from build123d import *

# Parameters (mm, degrees)
BOSS_EXTRU_1_DEPTH      = 4.35
ENL_V_MAT_EXTRU_1_DEPTH = 38.269393438
CONG_3_R                = 5
ESQUISSE3_R             = 1.5
ENL_V_MAT_EXTRU_2_DEPTH = 38.269393579
BOSS_EXTRU_2_DEPTH      = 4.35


with BuildPart() as part:
    # Esquisse1 → Boss.-Extru.1 (new body)
    with BuildSketch(Plane.XY):
        with BuildLine():
            Line((-13.183298291, -31.679408844), (-0.713739606, -32.039150948))
            ThreePointArc((-0.713739606, -32.039150948), (13.826896651, 2.211449904), (-6.128687986, 33.616997237))
            ThreePointArc((-6.128687986, 33.616997237), (-12.95399094, 31.768960554), (-11.105954257, 24.9436576))
            ThreePointArc((-11.105954257, 24.9436576), (3.84132079, 1.61453914), (-6.69721834, -24.00982412))
            ThreePointArc((-6.69721834, -24.00982412), (-10.263527106, -27.571231769), (-13.183298291, -31.679408844))
        make_face()
    extrude(amount=BOSS_EXTRU_1_DEPTH)

    # Esquisse2 → Enlèv. mat.-Extru.1 (cut, through all)
    with BuildSketch(Plane(origin=(0, 0, 0), x_dir=(-1, 0, 0), z_dir=(0, 0, -1))):
        with BuildLine():
            Line((13.183298291, -31.679408844), (0.713739606, -32.039150948))
            ThreePointArc((0.713739606, -32.039150948), (5.648573529, -29.472487497), (6.69721834, -24.00982412))
            ThreePointArc((6.69721834, -24.00982412), (10.263527106, -27.571231769), (13.183298291, -31.679408844))
        make_face()
    extrude(amount=-ENL_V_MAT_EXTRU_1_DEPTH, mode=Mode.SUBTRACT)

    # Congé3
    cong_3_edges = [part.edges().sort_by_distance(p)[0] for p in [
        (-0.713739606, -32.039150948, 2.175),
        (-6.69721834, -24.00982412, 2.175),
    ]]
    fillet(cong_3_edges, radius=CONG_3_R - 0.0001)  # a hair under: the kernel refuses the full size

    # Esquisse3 → Enlèv. mat.-Extru.2 (cut, through all)
    with BuildSketch(Plane.XY.offset(4.35)):
        with Locations((-8.617321121, 29.280327419)):
            Circle(ESQUISSE3_R)
        with Locations((8.901780596, 0.257662949)):
            Circle(ESQUISSE3_R)
        with Locations((-2.180082362, -26.639815256)):
            Circle(ESQUISSE3_R)
    extrude(amount=-ENL_V_MAT_EXTRU_2_DEPTH, mode=Mode.SUBTRACT)

    # Esquisse4 → Boss.-Extru.2 (add, through all)
    with BuildSketch(Plane.XY.offset(4.35)):
        with BuildLine():
            Line((-9.822535933, 22.144666991), (-8.891427789, 23.540777623))
            ThreePointArc((-8.891427789, 23.540777623), (-9.983360232, 24.266418144), (-11.105954257, 24.9436576))
            ThreePointArc((-11.105954257, 24.9436576), (-11.749605725, 25.383047193), (-12.317161418, 25.917117378))
            Line((-12.317161418, 25.917117378), (-12.247003841, 25.565996611))
            Line((-12.247003841, 25.565996611), (-11.635101494, 22.503581534))
            ThreePointArc((-11.635101494, 22.503581534), (-10.848728229, 21.718565469), (-9.822535933, 22.144666991))
        make_face()
        with BuildLine():
            Line((-6.720773728, 19.63604394), (-5.602744878, 20.887482618))
            ThreePointArc((-5.602744878, 20.887482618), (-7.081127932, 22.175442131), (-8.640486445, 23.364078822))
            Line((-8.640486445, 23.364078822), (-8.464930853, 20.246068108))
            ThreePointArc((-8.464930853, 20.246068108), (-7.796654849, 19.358351758), (-6.720773728, 19.63604394))
        make_face()
        with BuildLine():
            Line((-4.002247722, 16.716500355), (-2.719479126, 17.798439356))
            ThreePointArc((-2.719479126, 17.798439356), (-4.002235611, 19.281339204), (-5.379119408, 20.677278733))
            Line((-5.379119408, 20.677278733), (-5.643393478, 17.565531668))
            ThreePointArc((-5.643393478, 17.565531668), (-5.106472893, 16.592726743), (-4.002247722, 16.716500355))
        make_face()
        with BuildLine():
            Line((-1.720891689, 13.443958065), (-0.298832635, 14.33493243))
            ThreePointArc((-0.298832635, 14.33493243), (-1.360513504, 15.983352852), (-2.527606113, 17.558900694))
            Line((-2.527606113, 17.558900694), (-3.22646682, 14.515152299))
            ThreePointArc((-3.22646682, 14.515152299), (-2.831553807, 13.476558611), (-1.720891689, 13.443958065))
        make_face()
        with BuildLine():
            Line((0.078033764, 9.883342162), (1.611170559, 10.565675544))
            ThreePointArc((1.611170559, 10.565675544), (0.791628357, 12.346912961), (-0.142518712, 14.07081128))
            Line((-0.142518712, 14.07081128), (-1.262101119, 11.155447526))
            ThreePointArc((-1.262101119, 11.155447526), (-1.017030492, 10.071670094), (0.078033764, 9.883342162))
        make_face()
        with BuildLine():
            Line((1.358839136, 6.105292932), (2.972637242, 6.565448283))
            ThreePointArc((2.972637242, 6.565448283), (2.411492888, 8.444164113), (1.728824224, 10.282211897))
            Line((1.728824224, 10.282211897), (0.210731898, 7.553071689))
            ThreePointArc((0.210731898, 7.553071689), (0.301098098, 6.445611945), (1.358839136, 6.105292932))
        make_face()
        with BuildLine():
            Line((2.096114089, 2.184764392), (3.758556811, 2.413612532))
            ThreePointArc((3.758556811, 2.413612532), (3.46694304, 4.352534286), (3.04929648, 6.268265872))
            Line((3.04929648, 6.268265872), (1.16281219, 3.779493562))
            ThreePointArc((1.16281219, 3.779493562), (1.096681157, 2.670322781), (2.096114089, 2.184764392))
        make_face()
        with BuildLine():
            Line((2.275231572, -1.800462743), (3.953337136, -1.807462011))
            ThreePointArc((3.953337136, -1.807462011), (3.937039374, 0.15319873), (3.792700751, 2.108607261))
            Line((3.792700751, 2.108607261), (1.575251109, -0.090421541))
            ThreePointArc((1.575251109, -0.090421541), (1.35393484, -1.179298138), (2.275231572, -1.800462743))
        make_face()
        with BuildLine():
            Line((0.955923809, -9.649040634), (2.565827278, -10.122641832))
            ThreePointArc((2.565827278, -10.122641832), (3.095663042, -8.234857357), (3.501051982, -6.316494523))
            Line((3.501051982, -6.316494523), (0.759343223, -7.811768298))
            ThreePointArc((0.759343223, -7.811768298), (0.243820453, -8.79607994), (0.955923809, -9.649040634))
        make_face()
        with BuildLine():
            Line((1.89263801, -5.771324181), (3.553113903, -6.014031995))
            ThreePointArc((3.553113903, -6.014031995), (3.812455487, -4.07053049), (3.944288385, -2.114239038))
            Line((3.944288385, -2.114239038), (1.439866137, -3.979897042))
            ThreePointArc((1.439866137, -3.979897042), (1.067755401, -5.026876858), (1.89263801, -5.771324181))
        make_face()
        with BuildLine():
            Line((-0.516327235, -13.356680753), (1.011064381, -14.051779397))
            ThreePointArc((1.011064381, -14.051779397), (1.80088273, -12.257164359), (2.471785062, -10.414789202))
            Line((2.471785062, -10.414789202), (-0.452816504, -11.510013499))
            ThreePointArc((-0.452816504, -11.510013499), (-1.101523675, -12.412128869), (-0.516327235, -13.356680753))
        make_face()
        with BuildLine():
            Line((-2.494906628, -16.820687389), (-1.080329313, -17.723493178))
            ThreePointArc((-1.080329313, -17.723493178), (-0.046197856, -16.057651562), (0.876907606, -14.327815597))
            Line((0.876907606, -14.327815597), (-2.172564591, -15.001261883))
            ThreePointArc((-2.172564591, -15.001261883), (-2.941586238, -15.803283605), (-2.494906628, -16.820687389))
        make_face()
        with BuildLine():
            Line((-4.940560652, -19.972336923), (-3.666861923, -21.064938782))
            ThreePointArc((-3.666861923, -21.064938782), (-2.40893385, -19.560919792), (-1.251939064, -17.977941831))
            Line((-1.251939064, -17.977941831), (-4.365782364, -18.216249374))
            ThreePointArc((-4.365782364, -18.216249374), (-5.239861602, -18.902265862), (-4.940560652, -19.972336923))
        make_face()
        with BuildLine():
            ThreePointArc((-5.229503112, -22.686931264), (-4.539706777, -22.000844712), (-3.872520027, -21.292751794))
            Line((-3.872520027, -21.292751794), (-6.988957821, -21.091192728))
            ThreePointArc((-6.988957821, -21.091192728), (-7.95075349, -21.647593865), (-7.804769136, -22.749102695))
            Line((-7.804769136, -22.749102695), (-6.69721834, -24.00982412))
            ThreePointArc((-6.69721834, -24.00982412), (-5.952466431, -23.360464628), (-5.229503112, -22.686931264))
        make_face()
    extrude(amount=-BOSS_EXTRU_2_DEPTH)


solid = part.part
Model file for the job. Use its own axes, mm. A direction names the side the tool comes from. Give positions to 0.01 mm unless a question says otherwise; leave off trailing zeros. Order: outer loops, then holes, each group sorted by start corner. A loop starts at its lowest first (then second) coordinate and runs counter-clockwise, first axis right, second up. Notation, with made-up numbers: (16.25, 56.5) - (44.25, 56.5) arc R20 ccw to (44.25, 88.5) - close; hole circle Ø2 at (77.25, 43.25). An arc over 180 degrees is marked (long way). Write item = value, one per line. Start each with the question number.
1. Which spindle directions (+Z, -Z, +X, -X, +Y, -Y) get a long thin tool onto all of the face, cutting with end or side? Do faces 4 (the flat face through (0.98, 8.94, 2.21)), 5 (the flat face through (1.75, -9.883, 2.205)). Say none if no direction does.
2. Drop flat-ended pins along their axis: P1, Ø1.5, axis at x = 0, z = 2, coming from the +Y side; P2, Ø6, axis at x = 9.5, y = 21.5, coming from the +Z side; P3, Ø2, axis at x = -10, z = 1.5, coming from the +Y side; P4, Ø2.5, axis at x = 8.9, y = 0.26, coming from the +Z side. Give the stop position or say it passes through.
3. Two-plate mould, pull along Y, no slides. Class faces 1 (the flat face through (6, 2, 4.35)), 2 (the cylindrical face through (-1.029, 10.083, 2.205)), 3 (the cylindrical face through (13.72, 3.31, 2.14)): pulls with the +Y half, pulls with the -Y half, needs draft (parallel to the pull), parting line crosses it, or undercut.
4. Cut at A-A, the plane x = 9. List the corners of the cut face in (y, z), and give its area (3 significant figures).
5. Cut at D-D, the plane y = -7. List the corners of the cut face in (x, z), and give its area (3 significant figures).
6. Cut at B-B, the plane y = 30. List the corners of the cut face in (x, z), and give its area (3 significant figures).
7. Cut at C-C, the plane z = 2.5. State how many separate pieces and enclosed holes the cut face has, and give its area (3 significant figures).
8. Probe line 1 along Y through (x, z) = (-5, 1.85); line 2 along Y through (x, z) = (0.5, 0.8); line 3 along X through (y, z) = (10.5, 1.15). List the from-to ranges inside material, lowest first.
Taken from the geometry:
q1.face_4 = +Z, -Z
q1.face_5 = +Z, -Z, -X
q2.P1 = 29.92
q2.P2 = 4.35
q2.P3 = 34.27
q2.P4 = through
q3.face_1 = needs draft
q3.face_2 = undercut
q3.face_3 = parting line crosses it
q4.outline = (-20.37, 0) - (-1.24, 0) - (-1.24, 4.35) - (-20.37, 4.35) - close; (1.75, 0) - (18.22, 0) - (18.22, 4.35) - (1.75, 4.35) - close
q4.area = 155 mm²
q5.outline = (2.25, 0) - (13.52, 0) - (13.52, 4.35) - (2.25, 4.35) - close
q5.area = 49.0 mm²
q6.outline = (-13.57, 0) - (-9.93, 0) - (-9.93, 4.35) - (-13.57, 4.35) - close; (-7.3, 0) - (-0.85, 0) - (-0.85, 4.35) - (-7.3, 4.35) - close
q6.area = 43.8 mm²
q7.separate_pieces = 1
q7.enclosed_holes = 3
q7.area = 804 mm²
q8.line_1 = -30.1 to -21.22, -19.92 to -18.51, 16.55 to 32.94
q8.line_2 = -30.75 to -14.41, -13.82 to -11.15, -9.36 to -8.02, 6.26 to 8.07, 10.07 to 28.85
q8.line_3 = -1.28 to 1.46, 1.64 to 12.25
